Input: part model. Units: mm. Frame: model coordinates. A direction names the side the tool comes from. Coordinates: 2 decimals unless noted, no trailing zeros. Order: outer loops, then holes, each group sorted by start corner. A loop starts at its lowest first (then second) coordinate and runs counter-clockwise, first axis right, second up. Notation, with made-up numbers: M 65.5,-24 L 89.5,-24 A28 cw 89.5,-4 Z; hole C 43.5,-6 d4. An arc over 180 degrees is marked long. Answer in a Markdown table with one row per item.
from build123d import *

# Parameters (mm, degrees)
SCHIZZO1_W                   = 60
SCHIZZO1_H                   = 30
ESTRUSIONE_ESTRUSIONE1_DEPTH = 5
SCHIZZO2_W                   = 60
SCHIZZO2_H                   = 8
ESTRUSIONE_ESTRUSIONE2_DEPTH = 20
SCHIZZO3_R                   = 4.25
TAGLIO_ESTRUSIONE1_DEPTH     = 8
RACCORDO1_R                  = 20
SCHIZZO4_W                   = 60
SCHIZZO4_H                   = 15
ESTRUSIONE_ESTRUSIONE3_DEPTH = 10
SCHIZZO6_R                   = 8
TAGLIO_ESTRUSIONE2_DEPTH     = 15
SCHIZZO8_W                   = 60
SCHIZZO8_H                   = 4.5
ESTRUSIONE_ESTRUSIONE4_DEPTH = 10
SCHIZZO9_R                   = 6.3
TAGLIO_ESTRUSIONE3_DEPTH     = 4.5
SCHIZZO10_R                  = 2
TAGLIO_ESTRUSIONE4_DEPTH     = 16
SCHIZZO11_W                  = 60
SCHIZZO11_H                  = 15
TAGLIO_ESTRUSIONE5_DEPTH     = 1
SMUSSO1_SIZE                 = 0.5


with BuildPart() as part:
    # Schizzo1 → Estrusione-Estrusione1 (new body)
    with BuildSketch(Plane.XY):
        Rectangle(SCHIZZO1_W, SCHIZZO1_H)
    extrude(amount=ESTRUSIONE_ESTRUSIONE1_DEPTH)

    # Schizzo2 → Estrusione-Estrusione2 (add)
    with BuildSketch(Plane.XY.offset(5)):
        with Locations((0, 11)):
            Rectangle(SCHIZZO2_W, SCHIZZO2_H)
    extrude(amount=ESTRUSIONE_ESTRUSIONE2_DEPTH)

    # Schizzo3 → Taglio-Estrusione1 (cut)
    with BuildSketch(Plane(origin=(0, 15, 0), x_dir=(1, 0, 0), z_dir=(0, 1, 0))):
        with Locations((0, -13)):
            Circle(SCHIZZO3_R)
    extrude(amount=-TAGLIO_ESTRUSIONE1_DEPTH, mode=Mode.SUBTRACT)

    # Raccordo1
    raccordo1_edges = [part.edges().sort_by_distance(p)[0] for p in [
        (30, 11, 25),
        (-30, 11, 25),
    ]]
    fillet(raccordo1_edges, radius=RACCORDO1_R)

    # Schizzo4 → Estrusione-Estrusione3 (add)
    with BuildSketch(Plane.XY.offset(5)):
        with Locations((0, -0.5)):
            Rectangle(SCHIZZO4_W, SCHIZZO4_H)
    extrude(amount=ESTRUSIONE_ESTRUSIONE3_DEPTH)

    # Schizzo6 → Taglio-Estrusione2 (cut)
    with BuildSketch(Plane.XZ.offset(8)):
        with Locations((0, 13)):
            Circle(SCHIZZO6_R)
    extrude(amount=-TAGLIO_ESTRUSIONE2_DEPTH, mode=Mode.SUBTRACT)

    # Schizzo8 → Estrusione-Estrusione4 (add)
    with BuildSketch(Plane.XY.offset(15)):
        with Locations((0, -0.75)):
            Rectangle(SCHIZZO8_W, SCHIZZO8_H)
    extrude(amount=-ESTRUSIONE_ESTRUSIONE4_DEPTH)

    # Schizzo9 → Taglio-Estrusione3 (cut)
    with BuildSketch(Plane.XZ.offset(3)):
        with Locations((0, 13)):
            Circle(SCHIZZO9_R)
    extrude(amount=-TAGLIO_ESTRUSIONE3_DEPTH, mode=Mode.SUBTRACT)

    # Schizzo10 → Taglio-Estrusione4 (cut, through all)
    with BuildSketch(Plane.XY.offset(15)):
        with Locations((12, -0.85)):
            Circle(SCHIZZO10_R)
        with Locations((-12, -0.85)):
            Circle(SCHIZZO10_R)
    extrude(amount=-TAGLIO_ESTRUSIONE4_DEPTH, mode=Mode.SUBTRACT)

    # Schizzo11 → Taglio-Estrusione5 (cut)
    with BuildSketch(Plane.XY.offset(15)):
        with Locations((0, -0.5)):
            Rectangle(SCHIZZO11_W, SCHIZZO11_H)
    extrude(amount=-TAGLIO_ESTRUSIONE5_DEPTH, mode=Mode.SUBTRACT)

    # Smusso1
    smusso1_edges = [part.edges().sort_by_distance(p)[0] for p in [
        (-4.25, 15, 13),
    ]]
    chamfer(smusso1_edges, length=SMUSSO1_SIZE)


solid = part.part
1) Cut plane B-B, the plane z = 13. Output: boundary loops of the cut face in (x, y), and give its area (3 significant figures).
Resolved:
| item | result |
|---|---|
| outline | M -30,-8 L -8,-8 L -8,-3 L -6.3,-3 L -6.3,1.5 L -8,1.5 L -8,7 L -4.25,7 L -4.25,14.5 L -4.75,15 L -28.33,15 L -28.33,7 L -30,7 Z; M 4.25,7 L 8,7 L 8,1.5 L 6.3,1.5 L 6.3,-3 L 8,-3 L 8,-8 L 30,-8 L 30,7 L 28.33,7 L 28.33,15 L 4.75,15 L 4.25,14.5 Z; hole C -12,-0.85 d4; hole C 12,-0.85 d4 |
| area | 1,040 mm2 |
2) Mould query, pull axis Z, two halves, no side actions, for faces 5 (the face through (-0.15, -0.78, 6.7)), 6 (the face through (0, 0, 0)), 7 (the face through (-0.92, 10.8, 17.15)), 8 (the face through (18, -8, 9)). Classes: +Z half, -Z half, draft (parallel to the pull), parting line (faces both ways), or undercut.
Resolved:
| item | result |
|---|---|
| face 5 | undercut |
| face 6 | -Z half |
| face 7 | undercut |
| face 8 | draft |
3) Material intervals for probe 1 along Y at (x, z) = (-12, 9); probe 2 along Y at (x, z) = (12, 4); probe 3 along X at (y, z) = (0.45, 13), sorted ascending.
Resolved:
| item | result |
|---|---|
| probe 1 | y = -8 to -2.85, 1.15 to 15 |
| probe 2 | y = -15 to -2.85, 1.15 to 15 |
| probe 3 | x = -30 to -13.52, -10.48 to -6.3, 6.3 to 10.48, 13.52 to 30 |
4) Contact query for flat-ended pins moving along their axis: pin 1 (10 mm diameter, centred on x = -17, z = 10.5, fed in from -Y); pin 2 (2 mm diameter, centred on x = -14.5, y = -12.5, fed in from +Z); pin 3 (4.5 mm diameter, centred on x = -3, z = 11.5, fed in from -Y); pin 4 (5 mm diameter, centred on x = 0, z = 13, fed in from -Y). Output: stop coordinate, or through.
Resolved:
| item | result |
|---|---|
| pin 1 | stops at y = -8 |
| pin 2 | stops at z = 5 |
| pin 3 | stops at y = 7 |
| pin 4 | passes through |
5) Cut plane C-C, the plane x = 12. Output: boundary loops of the cut face in (y, z).
Resolved:
| item | result |
|---|---|
| outline | M -15,0 L -2.85,0 L -2.85,14 L -8,14 L -8,5 L -15,5 Z; M 1.15,0 L 15,0 L 15,24.9 L 7,24.9 L 7,14 L 1.15,14 Z |
6) Cut plane A-A, the plane y = -0.85. Output: boundary loops of the cut face in (x, z).
Resolved:
| item | result |
|---|---|
| outline | M -30,0 L -14,0 L -14,14 L -30,14 Z; M -10,0 L 10,0 L 10,14 L 6.22,14 A6.3 cw long -6.22,14 L -10,14 Z; M 14,0 L 30,0 L 30,14 L 14,14 Z |
7) Reachability of faces 1 (the face through (18, 0, 14)), 2 (the face through (0, -6, 5)), 3 (the face through (23.986, 11.056, 19.297)), 4 (the face through (30, 0, 5)) from +Z, -Z, +X, -X, +Y, -Y: full face, straight path, thin tool, end or side. Return the list, or none.
Resolved:
| item | result |
|---|---|
| face 1 | +Z, +X, -X, -Y |
| face 2 | -Y |
| face 3 | +Z, +X, +Y |
| face 4 | +Z, -Z, +X, +Y, -Y |
8) Cut plane D-D, the plane y = -10.75. Output: boundary loops of the cut face in (x, z), and give its area (3 significant figures).
Resolved:
| item | result |
|---|---|
| outline | M -30,0 L 30,0 L 30,5 L -30,5 Z |
| area | 300 mm2 |
